Check sheet for the modelled part. Datum: model origin and axes. Units: mm. Give positions to 0.01 mm unless a question says otherwise; leave off trailing zeros. Write each loop counter-clockwise with the first axis right and the second up, starting at its lowest first coordinate (ties: lowest second). Pieces come first, ordered by that corner, then holes. Notation, with made-up numbers: M 62.5,-40 L 70.5,-40 A29 ccw 70.5,-13 Z; hole C 27.5,77.5 d1. An arc over 180 degrees is marked long. Use CSV: the item, a comma, the result in double quotes. Start each with the question number.
1. Depth check by flat-ended pin: P1, Ø10, axis at x = 12, y = 109, coming from the +Z side; P2, Ø1, axis at y = 33.5, z = 1, coming from the -X side; P3, Ø1, axis at x = -2.5, z = 1.5, coming from the +Y side; P4, Ø0.6, axis at y = 228.5, z = 1, coming from the +X side. Enter the tip coordinate at first touch or a pass-through.
2. Scan lines: line 1 (Y direction, x = 33, z = 0.75); line 2 (Y direction, x = 28, z = 0.45); line 3 (X direction, y = 119, z = 1.85). Record each from-to range of solid material in increasing order.
3. Cross-section at A-A, the plane x = 13. Enter the section's corners in (y, z).
4. Cross-section at C-C, the plane y = 214.5. Enter the section's corners in (x, z), and give its area (3 significant figures).
5. Cross-section at B-B, the plane y = 113.5. Enter the section's corners in (x, z), and give its area (3 significant figures).
from build123d import *

# Parameters (mm, degrees)
SKETCH1_W               = 40
SKETCH1_H               = 227
BOSS_EXTRUDE1_DEPTH     = 2
SKETCH2_W               = 10
SKETCH2_H               = 2
BOSS_EXTRUDE2_DEPTH     = 3
LPATTERN1_COUNT         = 2
LPATTERN1_PITCH         = 20
SKETCH3_W               = 10
SKETCH3_H               = 2
BOSS_EXTRUDE3_DEPTH     = 3
LPATTERN2_COUNT         = 2
LPATTERN2_PITCH         = 20
SKETCH4_W               = 2
SKETCH4_H               = 10
BOSS_EXTRUDE4_DEPTH     = 3
LPATTERN3_COUNT         = 12
LPATTERN3_PITCH         = 20
ESQUISSE1_W             = 3
ESQUISSE1_H             = 3
ENL_V_MAT_EXTRU_1_DEPTH = 3
ESQUISSE2_W             = 1
ESQUISSE2_H             = 227
ESQUISSE2_W_2           = 43
ESQUISSE2_H_2           = 1
BOSS_EXTRU_1_DEPTH      = 2
ESQUISSE4_W             = 27
ESQUISSE4_H             = 45
ENL_V_MAT_EXTRU_2_DEPTH = 3


with BuildPart() as part:
    # Sketch1 → Boss-Extrude1 (new body)
    with BuildSketch(Plane.XY):
        with Locations((20, 113.5)):
            Rectangle(SKETCH1_W, SKETCH1_H)
    extrude(amount=BOSS_EXTRUDE1_DEPTH)

    # Sketch2 → Boss-Extrude2 (add)
    with BuildSketch(Plane.XZ):
        with Locations((25, 1)):
            Rectangle(SKETCH2_W, SKETCH2_H)
    boss_extrude2 = extrude(amount=BOSS_EXTRUDE2_DEPTH)

    # LPattern1: Boss-Extrude2 ×2
    with Locations(*[(-i * LPATTERN1_PITCH, 0, 0) for i in range(1, LPATTERN1_COUNT)]):
        add(boss_extrude2)

    # Sketch3 → Boss-Extrude3 (add)
    with BuildSketch(Plane(origin=(0, 227, 0), x_dir=(1, 0, 0), z_dir=(0, 1, 0))):
        with Locations((25, -1)):
            Rectangle(SKETCH3_W, SKETCH3_H)
    boss_extrude3 = extrude(amount=BOSS_EXTRUDE3_DEPTH)

    # LPattern2: Boss-Extrude3 ×2
    with Locations(*[(-i * LPATTERN2_PITCH, 0, 0) for i in range(1, LPATTERN2_COUNT)]):
        add(boss_extrude3)

    # Sketch4 → Boss-Extrude4 (add)
    with BuildSketch(Plane.ZY):
        with Locations((1, 5)):
            Rectangle(SKETCH4_W, SKETCH4_H)
    boss_extrude4 = extrude(amount=BOSS_EXTRUDE4_DEPTH)

    # LPattern3: Boss-Extrude4 ×12
    with Locations(*[(0, i * LPATTERN3_PITCH, 0) for i in range(1, LPATTERN3_COUNT)]):
        add(boss_extrude4)

    # Esquisse1 → Enlèv. mat.-Extru.1 (cut, through all)
    with BuildSketch(Plane.XY.offset(2)):
        with Locations((-1.5, 228.5)):
            Rectangle(ESQUISSE1_W, ESQUISSE1_H)
    extrude(amount=-ENL_V_MAT_EXTRU_1_DEPTH, mode=Mode.SUBTRACT)

    # Esquisse2 → Boss.-Extru.1 (add)
    with BuildSketch(Plane.XY.offset(2)):
        with Locations((-0.5, 113.5)):
            Rectangle(ESQUISSE2_W, ESQUISSE2_H)
        with Locations((18.5, -0.5)):
            Rectangle(ESQUISSE2_W_2, ESQUISSE2_H_2)
    extrude(amount=-BOSS_EXTRU_1_DEPTH)

    # Esquisse4 → Enlèv. mat.-Extru.2 (cut)
    with BuildSketch(Plane.XY.offset(2)):
        with Locations((20, 113)):
            Rectangle(ESQUISSE4_W, ESQUISSE4_H)
    extrude(amount=-ENL_V_MAT_EXTRU_2_DEPTH, mode=Mode.SUBTRACT)


solid = part.part
Worked answers:
1,P1,"passes through"
1,P2,"stops at x = -1"
1,P3,"stops at y = 227"
1,P4,"stops at x = 30"
2,line 1,"y = -1 to 90.5, 135.5 to 227"
2,line 2,"y = -3 to 90.5, 135.5 to 230"
2,line 3,"x = -1 to 6.5, 33.5 to 40"
3,outline,"M -1,0 L 90.5,0 L 90.5,2 L -1,2 Z; M 135.5,0 L 227,0 L 227,2 L 135.5,2 Z"
4,outline,"M -1,0 L 40,0 L 40,2 L -1,2 Z"
4,area,"82.0 mm^2"
5,outline,"M -1,0 L 6.5,0 L 6.5,2 L -1,2 Z; M 33.5,0 L 40,0 L 40,2 L 33.5,2 Z"
5,area,"28.0 mm^2"
